Autodesk Inventor part; units mm, degrees
ref_plane "YZ Plane" through (0, 0, 0) normal (1, 0, 0) x (0, 1, 0)
ref_plane "XZ Plane" through (0, 0, 0) normal (0, 1, 0) x (-1, 0, 0)
ref_plane "XY Plane" through (0, 0, 0) normal (0, 0, 1) x (1, 0, 0)
sketch "Sketch1" plane through (0, 0, 0) normal (0, 1, 0) x (-1, 0, 0)
  line L0 (0, 0) -> (150, 0)
  line L1 (150, 0) -> (150, -19.925)
  line L2 (150, -19.925) -> (0, -19.925)
  line L3 (0, -19.925) -> (0, 0)
  dimension "d0" = 150
  dimension "d1" = 19.925
extrude "Extrusion1" add sketch "Sketch1" along normal blind 4
sketch "Sketch2" plane through (0, 4, 0) normal (0, 1, 0) x (1, 0, 0)
  line L0 (-150, 0) -> (0, 0)
  line L1 (0, 19.925) -> (-150, 19.925)
  line L2 (0, 0) -> (-5, 0)
  line L3 (-5, 0) -> (-5, 19.925)
  line L4 (-5, 19.925) -> (0, 19.925)
  line L5 (0, 19.925) -> (0, 0)
  line L6 (-150.0001, 0) -> (-145.0001, 0)
  line L7 (-145.0001, 0) -> (-145.0001, 19.925)
  line L8 (-145.0001, 19.925) -> (-150.0001, 19.925)
  line L9 (-150.0001, 19.925) -> (-150.0001, 0)
  dimension "d4" = 5
  dimension "d5" = 5
extrude "Extrusion2" add sketch "Sketch2" along normal blind 12.175 contours L9 L1 L7 L0 | L3 L1 L5 L0
sketch "Sketch3" plane through (0, 4, 0) normal (0, 1, 0) x (1, 0, 0)
  line L0 (0, 19.925) -> (0, 0)
  line L1 (-150, 0) -> (-150, 19.925)
  line L2 (0, 19.925) -> (-150, 19.925)
  line L3 (-150, 19.925) -> (-150, 16.725)
  line L4 (-150, 16.725) -> (0, 16.725)
  line L5 (0, 16.725) -> (0, 19.925)
  dimension "d8" = 3.2
extrude "Extrusion3" add sketch "Sketch3" along normal blind 4.65
sketch "Sketch4" plane through (0, 4, 0) normal (0, 1, 0) x (1, 0, 0)
  line L0 (-5, 16.725) -> (-145.0001, 16.725) construction
  line L1 (-145.0001, 0) -> (-145.0001, 19.925) construction
  line L2 (-5, 16.725) -> (-145.0001, 16.725) construction
  line L3 (-145.0001, 16.725) -> (-145.0001, 6.225) construction
  line L4 (-145.0001, 6.225) -> (-5, 6.225) construction
  line L5 (-5, 6.225) -> (-5, 16.725) construction
  line L6 (-5, 19.925) -> (-5, 0)
  line L7 (-145.0001, 6.225) -> (-5, 6.225)
  line L8 (-5, 6.225) -> (-5, 3.475)
  line L9 (-5, 3.475) -> (-145.0001, 3.475)
  line L10 (-145.0001, 3.475) -> (-145.0001, 6.225)
  point P0 (0, 0)
  dimension "d11" = 10.5
  dimension "d12" = 2.75
extrude "Extrusion4" add sketch "Sketch4" along normal blind 3.5
sketch "Sketch5" plane through (-145.0001, 4, 0) normal (1, 0, 0) x (0, 0, -1)
  point P0 (0, -4)
sketch "Sketch6" plane through (-145.0001, 4, 0) normal (1, 0, 0) x (0, 0, -1)
  line L0 (6.225, 0) -> (16.725, 0) construction
  line L1 (16.725, 0) -> (16.725, -7.95) construction
  line L2 (16.725, -7.95) -> (6.225, -7.95) construction
  line L3 (6.225, -7.95) -> (6.225, 0) construction
  line L4 (6.225, 0) -> (16.725, 0) construction
  line L5 (16.725, 0) -> (16.725, 7.95) construction
  line L6 (16.725, 7.95) -> (6.225, 7.95) construction
  line L7 (6.225, 7.95) -> (6.225, 0) construction
  circle A0 centre (11.475, 7.95) radius 2.25
  point P0 (0, -4)
  dimension "d15" = 7.95
  dimension "d16" = 7.95
  dimension "d17" = 4.5
extrude "Extrusion5" cut sketch "Sketch6" along normal blind 155.75 and the other way blind 5.75
sketch "Sketch7" plane through (0, 4, 0) normal (0, 1, 0) x (1, 0, 0)
  line L0 (-145.0001, 3.475) -> (-145.0001, 0)
  line L1 (-145.0001, 3.475) -> (1.5965, 3.475)
  line L2 (1.5965, 3.475) -> (1.5965, -1.1679)
  line L3 (1.5965, -1.1679) -> (-145.0001, -1.1679)
  line L4 (-145.0001, -1.1679) -> (-145.0001, 3.475)
  line L5 (-145.0001, 3.475) -> (-5, 3.475)
  line L6 (-145.0001, 3.475) -> (-155.2913, 3.475)
  line L7 (-155.2913, 3.475) -> (-155.2913, -7.4286)
  line L8 (-155.2913, -7.4286) -> (-145.0001, -7.4286)
  line L9 (-145.0001, -7.4286) -> (-145.0001, 3.475)
  point P0 (0, 0)
extrude "Extrusion6" cut sketch "Sketch7" along normal blind 21 and the other way blind 34.875
sketch "Sketch8" plane through (0, 8.65, 0) normal (0, 1, 0) x (1, 0, 0)
  line L0 (-145.0001, 16.725) -> (-145.0001, 19.925) construction
  line L1 (-5, 16.725) -> (-145.0001, 16.725) construction
  line L2 (-145.0001, 19.925) -> (-5, 19.925) construction
  line L3 (-5, 19.925) -> (-5, 16.725) construction
  line L4 (-5, 16.725) -> (-145.0001, 16.725) construction
  line L5 (-145.0001, 16.725) -> (-145.0001, 19.925) construction
  line L6 (-150, 19.925) -> (0, 19.925)
  line L7 (-75, 19.925) -> (-70, 19.925)
  line L8 (-70, 19.925) -> (-70, 16.725)
  line L9 (-70, 16.725) -> (-75, 16.725)
  line L10 (-75, 16.725) -> (-75, 19.925)
  point P0 (0, 0)
  dimension "d26" = 5
extrude "Extrusion7" add sketch "Sketch8" along normal blind 3.8
fillet "Fillet1" radius 3 1 edges at (-70, 12.45, -18.325)
fillet "Fillet2" radius 3 1 edges at (-70, 8.65, -18.325)
sketch "Sketch9" plane through (0, 4, 0) normal (0, 1, 0) x (1, 0, 0)
  line L0 (-145.0001, 13.725) -> (-145.0001, 9.225) construction
  line L1 (-5, 9.225) -> (-5, 13.725) construction
  line L2 (-75.0001, 11.475) -> (-96.0001, 11.475) construction
  circle A0 centre (-96.0001, 11.475) radius 1.65
  line L3 (-75.0001, 11.475) -> (-54.0001, 11.475) construction
  circle A1 centre (-54.0001, 11.475) radius 1.65
  point P0 (0, 0)
  dimension "d33" = 21
  dimension "d34" = 3.3
  dimension "d35" = 21
  dimension "d36" = 3.3
extrude "Extrusion8" cut sketch "Sketch9" against normal blind 4
sketch "Sketch10" plane through (0, 4, 0) normal (0, 1, 0) x (1, 0, 0)
  circle A0 centre (-34, 11.475) radius 1.65 construction
  circle A1 centre (-34, 11.475) radius 1.65
  point P0 (0, 0)
  dimension "d39" = 3.3
extrude "Extrusion9" cut sketch "Sketch10" against normal blind 4
fillet "Fillet3" radius 2 3 edges at (-55.6501, 4, -11.475) (-35.65, 4, -11.475) (-97.6501, 4, -11.475)
sketch "Sketch11" plane through (0, 0, 0) normal (0, -1, 0) x (1, 0, 0)
  circle A0 centre (-96.0001, -11.475) radius 1.65 construction
  line L0 (-96.0001, -11.475) -> (-105.5001, -11.475) construction
  line L1 (-105.5, -8.75) -> (-105.5, -13.75)
  line L2 (-105.5, -13.75) -> (-117, -13.75)
  line L3 (-117, -13.75) -> (-117, -8.75)
  line L4 (-117, -8.75) -> (-105.5, -8.75)
  point P0 (0, 0)
  dimension "d43" = 9.5
  dimension "d44" = 5
  dimension "d45" = 11.5
extrude "Extrusion10" add sketch "Sketch11" along normal blind 9.5
sketch "Sketch12" plane through (-105.5, 0, -13.75) normal (0, 0, -1) x (-1, 0, 0)
  line L0 (0, -9.5) -> (11.5, -9.5) construction
  line L1 (0, 0) -> (11.5, 0) construction
  line L2 (11.5, -9.5) -> (0, 0) construction
  line L3 (0, 0) -> (0, -9.5) construction
  line L4 (0, -9.5) -> (11.5, 0) construction
  circle A0 centre (5.75, -4.75) radius 2
  line L5 (11.5, -9.5) -> (0, -9.5)
  line L6 (0, -9.5) -> (0, 0)
  line L7 (0, 0) -> (11.5, 0)
  line L8 (11.5, 0) -> (11.5, -9.5)
  point P0 (-105.5, 0)
  dimension "d48" = 4
sketch "Sketch13" plane through (-105.5, 0, -13.75) normal (0, 0, -1) x (-1, 0, 0)
  point P0 (-105.5, 0)
extrude "Extrusion11" add sketch "Sketch12" along normal blind 6.175
sketch "Sketch14" plane through (-111.25, -4.75, -13.75) normal (0, 0, -1) x (-1, 0, 0)
  circle A0 centre (0, 0) radius 2
  point P0 (-111.25, 4.75)
extrude "Extrusion12" cut sketch "Sketch14" against normal blind 1.825
sketch "Sketch15" plane through (-111.25, -4.75, -11.925) normal (0, 0, -1) x (-1, 0, 0)
  circle A0 centre (0, 0) radius 2
  point P0 (-111.25, 4.75)
extrude "Extrusion13" cut sketch "Sketch15" against normal blind 0.5
sketch "Sketch16" plane through (-105.5, 0, -19.925) normal (0, 0, -1) x (-1, 0, 0)
  point P0 (-105.5, 0)
sketch "Sketch17" plane through (0, 0, 0) normal (0, -1, 0) x (1, 0, 0)
  point P0 (0, 0)
sketch "Sketch18" plane through (-111.25, -4.75, -11.425) normal (0, 0, -1) x (-1, 0, 0)
  circle A0 centre (0, 0) radius 2
  circle A1 centre (0, 0) radius 2
  point P0 (-111.25, 4.75)
extrude "Extrusion14" add sketch "Sketch18" along normal blind 4.5
sketch "Sketch19" plane through (0, -9.5, 0) normal (0, -1, 0) x (1, 0, 0)
  line L0 (-105.5, -8.75) -> (-117, -8.75)
  line L1 (-105.5, -8.75) -> (-105.5, -19.925)
  line L2 (-117, -8.75) -> (-105.5, -8.75)
  line L3 (-105.5, -8.75) -> (-105.5, -12.75)
  line L4 (-105.5, -12.75) -> (-117, -12.75)
  line L5 (-117, -12.75) -> (-117, -8.75)
  point P0 (0, 0)
  dimension "d57" = 4
extrude "Extrusion15" cut sketch "Sketch19" against normal blind 9.5
sketch "Sketch20" plane through (-117, -9.5, -12.75) normal (0, 0, 1) x (1, 0, 0)
  line L0 (11.5, 9.5) -> (11.5, 0) construction
  line L1 (0, 0) -> (0, 9.5) construction
  line L2 (11.5, 9.5) -> (0, 9.5) construction
  line L3 (0, 9.5) -> (0, 2) construction
  line L4 (0, 2) -> (11.5, 2) construction
  line L5 (11.5, 2) -> (11.5, 9.5) construction
  line L6 (-33, 9.5) -> (0, 9.5) construction
  line L7 (11.5, 2) -> (0, 9.5) construction
  line L8 (0, 9.5) -> (0, 2) construction
  line L9 (11.5, 9.5) -> (0, 2) construction
  line L10 (5.75, 5.75) -> (2.87, 5.75) construction
  line L11 (5.75, 5.75) -> (8.63, 5.75) construction
  circle A0 centre (8.63, 5.75) radius 1.5
  circle A1 centre (2.87, 5.75) radius 1.5
  point P0 (117, 9.5)
  dimension "d60" = 7.5
  dimension "d61" = 2.88
  dimension "d62" = 2.88
  dimension "d63" = 3
  dimension "d64" = 3
extrude "Extrusion16" add sketch "Sketch20" along normal blind 2.5
sketch "Sketch21" plane through (0, 16.175, -19.925) normal (0, 0, -1) x (-1, 0, 0)
  line L0 (0, -16.175) -> (150, -16.175)
  line L1 (105.5, -16.175) -> (117, -16.175)
  line L2 (117, -16.175) -> (117, -13.675)
  line L3 (117, -13.675) -> (105.5, -13.675)
  line L4 (105.5, -13.675) -> (105.5, -16.175)
  dimension "d67" = 2.5
extrude "Extrusion17" add sketch "Sketch21" along normal blind 3
sketch "Sketch22" plane through (-117, 2.5, -19.925) normal (0, 1, 0) x (1, 0, 0)
  line L0 (0, 3) -> (11.5, 3)
  line L1 (0, 0) -> (0, 3)
  line L2 (11.5, 3) -> (0, 3)
  line L3 (0, 3) -> (0, 1)
  line L4 (0, 1) -> (11.5, 1)
  line L5 (11.5, 1) -> (11.5, 3)
  point P0 (117, -19.925)
  dimension "d70" = 2
extrude "Extrusion18" add sketch "Sketch22" along normal blind 2.5
fillet "Fillet4" radius 1 2 edges at (-117, 3.75, -20.925) (-105.5, 3.75, -20.925)
equation "\"BendRadius\" = Thickness"
equation "\"BendReliefWidth\" = Thickness"
equation "\"BendReliefDepth\" = 0.5 * Thickness"
equation "\"CornerReliefSize\" = 4 * Thickness"
equation "\"MinimumRemnant\" = 2 * Thickness"
equation "\"TransitionRadius\" = BendRadius"
equation "\"JacobiRadiusSize\" = BendRadius"
equation "\"GapSize\" = Thickness"
properties part number "mtv_axelHolder(brakingAxel)3-12"
Read the model definition and answer for the solid it produces. Units are mm, in the model's axes. A direction names the side the tool comes from. Coordinates: 2 decimals unless noted, no trailing zeros. Order: outer loops, then holes, each group sorted by start corner. A loop starts at its lowest first (then second) coordinate and runs counter-clockwise, first axis right, second up. Notation, with made-up numbers: (51, 78) -> (67, 78) arc R21 ccw to (67, 117) -> close; hole circle Ø4 at (48, 78). An arc over 180 degrees is marked (long way). Answer as a JSON object with one key per item and string values.
1) Consider line 1 along X through (y, z) = (7, -11.75); line 2 along Z through (x, y) = (-124, 4.75) (3 decimals); line 3 along Y through (x, z) = (-111.25, -19.05). Determine where each line is inside the solid, lowest interval first. Write a range as from..to.
Model answer:
{"line 1": "x = -150..-145, -5..0", "line 2": "z = -19.925..-16.725, -6.225..-3.475", "line 3": "y = -9.5..-6.75, -2.75..8.65"}
2) A cutting plane is placed at B-B, the plane x = -111.25. Determine the outline of the cut face in (y, z) (3 decimals), plus the area to 3 significant figures.
Model answer:
{"outline": "(-9.5, -19.925) -> (-6.75, -19.925) -> (-6.75, -15.925) -> (-2.75, -15.925) -> (-2.75, -19.925) -> (0, -19.925) -> (0, -22.925) -> (5, -22.925) -> (5, -20.925) -> (2.5, -20.925) -> (2.5, -19.925) -> (8.65, -19.925) -> (8.65, -16.725) -> (4, -16.725) -> (4, -6.225) -> (7.5, -6.225) -> (7.5, -3.475) -> (0, -3.475) -> (0, -12.75) -> (-9.5, -12.75) -> close", "area": "155 mm²"}
3) Each of these flat-tipped pins is pushed along its axis until it touches: pin 1 (6 mm diameter, centred on y = 8, z = -10.5, fed in from +X); pin 2 (2 mm diameter, centred on x = -114, z = -22.5, fed in from +Y); pin 3 (5 mm diameter, centred on x = -93, y = 2.5, fed in from -Z) (3 decimals); pin 4 (5 mm diameter, centred on x = -111.25, y = -4.75, fed in from +Z). Where does it stop, or does it pass through?
Model answer:
{"pin 1": "stops at x = 0", "pin 2": "stops at y = 5", "pin 3": "stops at z = -19.925", "pin 4": "stops at z = -10.25"}
4) A cutting plane is placed at A-A, the plane x = -39.5. Determine the outline of the cut face in (y, z) (3 decimals).
Model answer:
{"outline": "(0, -19.925) -> (8.65, -19.925) -> (8.65, -16.725) -> (4, -16.725) -> (4, -6.225) -> (7.5, -6.225) -> (7.5, -3.475) -> (0, -3.475) -> close"}
5) The mould has two halves that part along X. Classify faces 6 (the face through (-117, -5, -16)), 7 (the face through (-111, -5, -15.925)), 8 (the face through (0, 8, -12)): released by +X, released by -X, zero draft, split by the parting line, or undercut.
Model answer:
{"face 6": "released by -X", "face 7": "undercut", "face 8": "released by +X"}
6) A tool of negligible diameter and unlimited length cuts with its end or side. For faces 1 (the face through (-114, -4, -10.25)), 2 (the face through (-74, 4, -11)), 3 (the face through (-76, 7.5, -5)), 4 (the face through (-109.252, -4.838, -17.897)), 5 (the face through (-115.63, -3.82, -11.52)), from which of +Z, -Z, +X, -X, +Y, -Y can it reach the whole face along a straight path? Write none if from no direction.
Model answer:
{"face 1": "+Z, +X, -X, -Y", "face 2": "+Y", "face 3": "+Z, +Y", "face 4": "-Z", "face 5": "+Z"}
